```python
from build123d import *

# Parameters (mm, degrees)
F0_R     = 15
F1_DEPTH = 3.95
F2_R     = 7.375
F2_R_2   = 5.375
F3_DEPTH = 16
F4_W     = 23.3622987423
F4_H     = 4
F5_DEPTH = 13.5
F6_R     = 1


with BuildPart() as f1:
    # F0 (on Top) → F1 (new body)
    with BuildSketch(Plane.XY):
        Circle(F0_R)
    extrude(amount=F1_DEPTH)

    # F2 (on face) → F3 (join)
    with BuildSketch(Plane.XY.offset(3.95)):
        Circle(F2_R)
        Circle(F2_R_2, mode=Mode.SUBTRACT)
    extrude(amount=F3_DEPTH)

    # F4 (on face) → F5 (cut, through all)
    with BuildSketch(Plane.XY.offset(19.95)):
        Rectangle(F4_W, F4_H)
    extrude(amount=-F5_DEPTH, mode=Mode.SUBTRACT)

    # F6
    f6_edges = [f1.edges().sort_by_distance(p)[0] for p in [
        (0, -7.375, 19.95),
        (0, 7.375, 19.95),
        (15, 0, 1.975),
        (-15, 0, 0),
        (-15, 0, 3.95),
    ]]
    fillet(f6_edges, radius=F6_R)


solid = f1.part
```
Geometry: final body of the model. Coordinates: model frame, mm. A direction names the side the tool comes from. Coordinates: 2 decimals unless noted, no trailing zeros. Order: outer loops, then holes, each group sorted by start corner. A loop starts at its lowest first (then second) coordinate and runs counter-clockwise, first axis right, second up. Notation, with made-up numbers: (74, -31) -> (133, -31) arc R23 ccw to (133, -18) -> close; hole circle Ø1 at (11.25, 4.5). An arc over 180 degrees is marked (long way). Write item = value, one per line.
(1) Line query: line 1 (Y direction, x = 0, z = 9) (3 decimals); line 2 (Z direction, x = -12, y = 0.5); line 3 (Z direction, x = 6.75, y = -1). Output: solid intervals per line, ascending.
Solved:
line_1 = -7.375 to -5.375, 5.375 to 7.375
line_2 = 0 to 3.95
line_3 = 0 to 6.45
(2) Access query for faces 5 (the flat face through (0, -6, 19.95)), 6 (the flat face through (6, 2, 13)), 7 (the cylindrical face through (-1.165, -5.247, 11.838)). Directions: +Z, -Z, +X, -X, +Y, -Y. A direction counts if a zero-diameter tool reaches every point of the face in a straight line with its end or side. Return the directions, or none.
Solved:
face_5 = +Z, +X, -X, +Y, -Y
face_6 = +Z, +X, -X
face_7 = +Z
(3) Pull-direction query (Y, two-part tool) for faces 1 (the flat face through (0, 0, 3.95)), 2 (the flat face through (-6, 0, 6.45)), 3 (the flat face through (0, 0, 0)), 4 (the cylindrical face through (7.034, 2.215, 11.345)); classes: pulls with the +Y half, pulls with the -Y half, needs draft (parallel to the pull), parting line crosses it, or undercut.
Solved:
face_1 = undercut
face_2 = undercut
face_3 = needs draft
face_4 = parting line crosses it
(4) Cut plane B-B on x = 0. Return loops of the section in (y, z) (3 decimals).
Solved:
outline = (-15, 1) arc R1 ccw to (-14, 0) -> (14, 0) arc R1 ccw to (15, 1) -> (15, 2.95) arc R1 ccw to (14, 3.95) -> (7.375, 3.95) -> (7.375, 18.95) arc R1 ccw to (6.375, 19.95) -> (5.375, 19.95) -> (5.375, 3.95) -> (-5.375, 3.95) -> (-5.375, 19.95) -> (-6.375, 19.95) arc R1 ccw to (-7.375, 18.95) -> (-7.375, 3.95) -> (-14, 3.95) arc R1 ccw to (-15, 2.95) -> close
(5) Cut plane A-A on z = 14.5. Return loops of the section in (x, y) (3 decimals).
Solved:
outline = (-7.099, -2) arc R7.375 ccw to (7.099, -2) -> (4.989, -2) arc R5.375 cw to (-4.989, -2) -> close; (-7.099, 2) -> (-4.989, 2) arc R5.375 cw to (4.989, 2) -> (7.099, 2) arc R7.375 ccw to start
(6) Cut plane C-C on y = 0. Return loops of the section in (x, z) (3 decimals).
Solved:
outline = (-15, 1) arc R1 ccw to (-14, 0) -> (14, 0) arc R1 ccw to (15, 1) -> (15, 2.95) arc R1 ccw to (14, 3.95) -> (7.375, 3.95) -> (7.375, 6.45) -> (5.375, 6.45) -> (5.375, 3.95) -> (-5.375, 3.95) -> (-5.375, 6.45) -> (-7.375, 6.45) -> (-7.375, 3.95) -> (-14, 3.95) arc R1 ccw to (-15, 2.95) -> close
(7) Cut plane D-D on z = 1.75. Return loops of the section in (x, y), plus the area to 3 significant figures.
Solved:
outline = circle Ø30 at (0, 0)
area = 707 mm²
(8) Pin query (flat end, axial travel): pin 1 Ø5 at (x, z) = (11.5, 11.5) entering from +Y; pin 2 Ø1 at (x, y) = (2.5, -2) entering from +Z; pin 3 Ø1 at (x, z) = (6.5, 7.5) entering from +Y; pin 4 Ø1.1 at (x, z) = (-5.5, 16.5) entering from -Y. Return the tip coordinate at first contact, or that it passes through.
Solved:
pin_1 = through
pin_2 = 3.95
pin_3 = 4.29
pin_4 = -5.47
